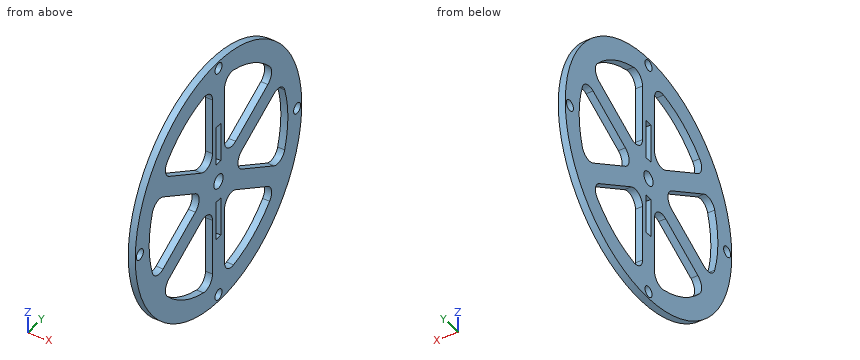
from build123d import *

# Parameters (mm, degrees)
SKETCH1_R              = 57.15
SKETCH1_W              = 17.78
SKETCH1_H              = 3.302
BOSS_EXTRUDE1_DEPTH    = 3.175
CUT_EXTRUDE1_START     = -3.175
CUT_EXTRUDE1_OUTLINE_R = 3.175
CUT_EXTRUDE1_DEPTH     = 3.175
F_10_24_TAPPED_HOLE1_D = 4.826


# Read off the part's stored shape, not the designer's step: Cut-Extrude1
with BuildPart() as part:
    # Sketch1 → Boss-Extrude1 (new body)
    with BuildSketch(Plane(origin=(0, 0, 0), x_dir=(0, 0, -1), z_dir=(1, 0, 0))):
        Circle(SKETCH1_R)
        with Locations((-17.78, 0)):
            Rectangle(SKETCH1_W, SKETCH1_H, mode=Mode.SUBTRACT)
        with Locations((17.78, 0)):
            Rectangle(SKETCH1_W, SKETCH1_H, mode=Mode.SUBTRACT)
    extrude(amount=BOSS_EXTRUDE1_DEPTH)

    # Cut-Extrude1 outline → Cut-Extrude1 (cut)
    with BuildSketch(Plane(origin=(3.175, 0, 0), x_dir=(0, 0, -1), z_dir=(1, 0, 0)).offset(CUT_EXTRUDE1_START)):
        with BuildLine():
            Line((-17.193839306, 38.035603254), (-4.399409051, 15.875))
            ThreePointArc((-4.399409051, 15.875), (0, 13.335), (4.399409051, 15.875))
            Line((4.399409051, 15.875), (17.193839306, 38.035603254))
            ThreePointArc((17.193839306, 38.035603254), (17.529050695, 42.416735863), (14.322123419, 45.420451404))
            ThreePointArc((14.322123419, 45.420451404), (0, 47.625), (-14.322123419, 45.420451404))
            ThreePointArc((-14.322123419, 45.420451404), (-17.529050695, 42.416735863), (-17.193839306, 38.035603254))
        make_face()
        with BuildLine():
            ThreePointArc((15.947857811, -4.1275), (11.548448759, -6.6675), (11.548448759, -11.7475))
            Line((11.548448759, -11.7475), (24.342879014, -33.908103254))
            ThreePointArc((24.342879014, -33.908103254), (27.969445455, -36.388971138), (32.174203058, -35.113548419))
            ThreePointArc((32.174203058, -35.113548419), (41.244459855, -23.8125), (46.496326477, -10.306902985))
            ThreePointArc((46.496326477, -10.306902985), (45.49849615, -6.027764725), (41.536718319, -4.1275))
            Line((41.536718319, -4.1275), (15.947857811, -4.1275))
        make_face()
        with BuildLine():
            ThreePointArc((-24.342879014, 33.908103254), (-27.969445455, 36.388971138), (-32.174203058, 35.113548419))
            ThreePointArc((-32.174203058, 35.113548419), (-41.244459855, 23.8125), (-46.496326477, 10.306902985))
            ThreePointArc((-46.496326477, 10.306902985), (-45.49849615, 6.027764725), (-41.536718319, 4.1275))
            Line((-41.536718319, 4.1275), (-15.947857811, 4.1275))
            ThreePointArc((-15.947857811, 4.1275), (-11.548448759, 6.6675), (-11.548448759, 11.7475))
            Line((-11.548448759, 11.7475), (-24.342879014, 33.908103254))
        make_face()
        with BuildLine():
            ThreePointArc((-41.536718319, -4.1275), (-45.49849615, -6.027764725), (-46.496326477, -10.306902985))
            ThreePointArc((-46.496326477, -10.306902985), (-41.244459855, -23.8125), (-32.174203058, -35.113548419))
            ThreePointArc((-32.174203058, -35.113548419), (-27.969445455, -36.388971138), (-24.342879014, -33.908103254))
            Line((-24.342879014, -33.908103254), (-11.548448759, -11.7475))
            ThreePointArc((-11.548448759, -11.7475), (-11.548448759, -6.6675), (-15.947857811, -4.1275))
            Line((-15.947857811, -4.1275), (-41.536718319, -4.1275))
        make_face()
        with BuildLine():
            ThreePointArc((-17.193839306, -38.035603254), (-17.529050695, -42.416735863), (-14.322123419, -45.420451404))
            ThreePointArc((-14.322123419, -45.420451404), (0, -47.625), (14.322123419, -45.420451404))
            ThreePointArc((14.322123419, -45.420451404), (17.529050695, -42.416735863), (17.193839306, -38.035603254))
            Line((17.193839306, -38.035603254), (4.399409051, -15.875))
            ThreePointArc((4.399409051, -15.875), (0, -13.335), (-4.399409051, -15.875))
            Line((-4.399409051, -15.875), (-17.193839306, -38.035603254))
        make_face()
        with BuildLine():
            ThreePointArc((41.536718319, 4.1275), (45.49849615, 6.027764725), (46.496326477, 10.306902985))
            ThreePointArc((46.496326477, 10.306902985), (41.244459855, 23.8125), (32.174203058, 35.113548419))
            ThreePointArc((32.174203058, 35.113548419), (27.969445455, 36.388971138), (24.342879014, 33.908103254))
            Line((24.342879014, 33.908103254), (11.548448759, 11.7475))
            ThreePointArc((11.548448759, 11.7475), (11.548448759, 6.6675), (15.947857811, 4.1275))
            Line((15.947857811, 4.1275), (41.536718319, 4.1275))
        make_face()
        Circle(CUT_EXTRUDE1_OUTLINE_R)
    extrude(amount=CUT_EXTRUDE1_DEPTH, mode=Mode.SUBTRACT)

    # #10-24 Tapped Hole1 (through all)
    with Locations(Plane(origin=(3.175, 0, 0), x_dir=(0, 0, -1), z_dir=(1, 0, 0))):
        with Locations((-53.975, 0), (0, 53.975), (53.975, 0), (0, -53.975)):
            Hole(F_10_24_TAPPED_HOLE1_D / 2)


solid = part.part
Check sheet for the modelled part. Datum: model origin and axes. Units: mm. Give positions to 0.01 mm unless a question says otherwise; leave off trailing zeros. Loops run counter-clockwise (first coordinate to the right, second up) from the corner with the lowest first, then second, coordinate; pieces in that order, holes last. Notation, with made-up numbers: M 8.5,-2 L 53.5,-2 A25 ccw 53.5,17 Z; hole C 82,72.25 d11. An arc over 180 degrees is marked long. Return JSON: item names as keys, results as strings. Group by question number.
1. Cross-section at B-B on y = 0. Record the boundary of the cut face in (x, z) (3 decimals), plus the area to 3 significant figures.
2. Go/stop test with flat-tipped pins: pin 1 (1.6 mm diameter, centred on x = 1.5, z = -17.5, fed in from -Y); pin 2 (1.6 mm diameter, centred on x = 2, z = 20.5, fed in from +Y); pin 3 (1 mm diameter, centred on x = 2.5, z = 13.5, fed in from -Y); pin 4 (5.5 mm diameter, centred on y = -53.975, z = 0, fed in from +X) (3 decimals). Record where each tip stops, or that it passes through.
3. Cross-section at C-C on y = 29. Record the boundary of the cut face in (x, z) (3 decimals), plus the area to 3 significant figures.
4. Cross-section at A-A on z = 0. Record the boundary of the cut face in (x, y) (3 decimals), plus the area to 3 significant figures.
5. Cross-section at D-D on x = 2. State how many separate pieces and enclosed holes the cut face has, plus the area to 3 significant figures.
6. Thickness scan on L1, parallel to Y at x = 2.6, z = -17; L2, parallel to Y at x = 2.4, z = 19.5; L3, parallel to Y at x = 0.6, z = -10. Record the ranges inside material, lowest first.
Return value:
{
 "1": {"outline": "M 0,-57.15 L 3.175,-57.15 L 3.175,-56.388 L 0,-56.388 Z; M 0,-51.562 L 3.175,-51.562 L 3.175,-26.67 L 0,-26.67 Z; M 0,-8.89 L 3.175,-8.89 L 3.175,-3.175 L 0,-3.175 Z; M 0,3.175 L 3.175,3.175 L 3.175,8.89 L 0,8.89 Z; M 0,26.67 L 3.175,26.67 L 3.175,51.562 L 0,51.562 Z; M 0,56.388 L 3.175,56.388 L 3.175,57.15 L 0,57.15 Z", "area": "199 mm^2"},
 "2": {"pin 1": "y = -54.66", "pin 2": "y = 53.65", "pin 3": "y = -55.65", "pin 4": "x = 3.175"},
 "3": {"outline": "M 0,-49.246 L 3.175,-49.246 L 3.175,-37.778 L 0,-37.778 Z; M 0,-21.509 L 3.175,-21.509 L 3.175,-11.977 L 0,-11.977 Z; M 0,11.977 L 3.175,11.977 L 3.175,21.509 L 0,21.509 Z; M 0,37.778 L 3.175,37.778 L 3.175,49.246 L 0,49.246 Z", "area": "133 mm^2"},
 "4": {"outline": "M 0,-57.15 L 3.175,-57.15 L 3.175,-56.388 L 0,-56.388 Z; M 0,-51.562 L 3.175,-51.562 L 3.175,-47.625 L 0,-47.625 Z; M 0,-13.335 L 3.175,-13.335 L 3.175,-3.175 L 0,-3.175 Z; M 0,3.175 L 3.175,3.175 L 3.175,13.335 L 0,13.335 Z; M 0,47.625 L 3.175,47.625 L 3.175,51.562 L 0,51.562 Z; M 0,56.388 L 3.175,56.388 L 3.175,57.15 L 0,57.15 Z", "area": "94.4 mm^2"},
 "5": {"separate pieces": "1", "enclosed holes": "13", "area": "5,300 mm^2"},
 "6": {"L1": "-54.56 to -43.43, -37.7 to -21.19, -4.13 to -1.65, 1.65 to 4.13, 21.19 to 37.7, 43.43 to 54.56", "L2": "-53.72 to -25.52, -4.13 to -1.65, 1.65 to 4.13, 25.52 to 53.72", "L3": "-56.27 to -46.56, -25.58 to -1.65, 1.65 to 25.58, 46.56 to 56.27"}
}
